The model under review builds one solid part; all positions refer to its coordinate system, in mm. Round coordinates to 2 decimals unless told otherwise and drop trailing zeros. Loops run counter-clockwise (first coordinate to the right, second up) from the corner with the lowest first, then second, coordinate; pieces in that order, holes last. Notation, with made-up numbers: M -16.75,20.5 L -7.75,20.5 A15 cw -7.75,48.5 Z; hole C -17.75,50 d4. An arc over 180 degrees is marked long. Return JSON: item names as keys, results as strings. Group by question number.
Q1. To check wall thickness, follow line 1 along Z through (x, y) = (3.5, 0.5); line 2 along Z through (x, y) = (5, 1.75); line 3 along X through (y, z) = (1.75, 18.75). State the ranges of each line that lie inside material, in increasing order.
Q2. Clearance check with flat-ended pins moving along their axes: pin 1 Ø1.5 at (x, y) = (6, 6) entering from +Z; pin 2 Ø2 at (y, z) = (4, 16) entering from -X; pin 3 Ø10 at (x, z) = (5.5, 6) entering from -Y; pin 4 Ø3 at (x, y) = (4.5, 3.5) entering from +Z. State where each tip first meets the part, or that it passes through.
Q3. Consider section B-B (z = 23). State the section outline as (x, y) points, and give its area (3 significant figures).
Q4. Consider section A-A (y = 5). State the section outline as (x, z) points, and give its area (3 significant figures).
Q5. Consider section C-C (x = 4.5). State the section outline as (y, z) points, and give its area (3 significant figures).
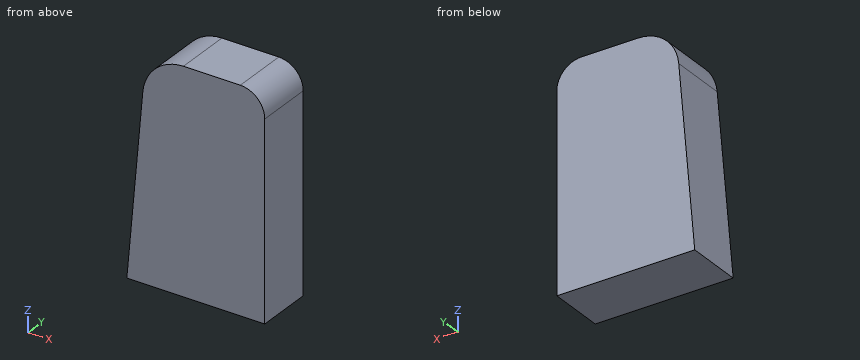
from build123d import *

# Parameters (mm, degrees)
BOX_W               = 20
BOX_H               = 20
BOX_DEPTH           = 40
BOX_PLACEMENT_ANGLE = 5
BOX001_W            = 17
BOX001_H            = 7
BOX001_DEPTH        = 27
FILLET_R            = 5
FILLET001_R         = 3


with BuildPart() as cube:
    # Box → Box (new body)
    with BuildSketch(Plane.XY):
        with Locations((10, 10)):
            Rectangle(BOX_W, BOX_H)
    extrude(amount=BOX_DEPTH)


with BuildPart() as cube_1:
    # Box placement: moved
    add(cube.part.moved(Location((-20, 0, 0))).rotate(Axis((-20, 0, 0), (0, 1, 0)), BOX_PLACEMENT_ANGLE))


with BuildPart() as fillet001:
    # Box001 → Box001 (new body)
    with BuildSketch(Plane.XY):
        with Locations((8.5, 3.5)):
            Rectangle(BOX001_W, BOX001_H)
    extrude(amount=BOX001_DEPTH)

    # Cut: cut Cube
    add(cube_1.part, mode=Mode.SUBTRACT)

    # Fillet
    fillet_edges = [fillet001.edges().sort_by_distance(p)[0] for p in [
        (2.438591, 3.5, 27),
    ]]
    fillet(fillet_edges, radius=FILLET_R)

    # Fillet001
    fillet001_edges = [fillet001.edges().sort_by_distance(p)[0] for p in [
        (17, 3.5, 27),
    ]]
    fillet(fillet001_edges, radius=FILLET001_R)


solid = fillet001.part
Values:
{
 "1": {"line 1": "z = 0 to 25.55", "line 2": "z = 0 to 26.57", "line 3": "x = 1.72 to 17"},
 "2": {"pin 1": "stops at z = 26.99", "pin 2": "stops at x = 1.39", "pin 3": "stops at y = 0", "pin 4": "stops at z = 26.89"},
 "3": {"outline": "M 2.12,0 L 17,0 L 17,7 L 2.12,7 Z", "area": "104 mm2"},
 "4": {"outline": "M 0.08,0 L 17,0 L 17,24 A3 ccw 14,27 L 7.02,27 A5 ccw 2.04,22.44 Z", "area": "419 mm2"},
 "5": {"outline": "M 0,0 L 7,0 L 7,26.32 L 0,26.32 Z", "area": "184 mm2"}
}
